Source: CAD feature listing. Evaluate the final solid. Frame: model axes, mm. Give positions to 0.01 mm unless a question says otherwise; leave off trailing zeros. Order: outer loops, then holes, each group sorted by start corner. A loop starts at its lowest first (then second) coordinate and runs counter-clockwise, first axis right, second up. Notation, with made-up numbers: (11.25, 3) - (26.25, 3) arc R13 cw to (26.25, 28) - close; hole circle Ø3 at (-7.5, 32.25). An arc over 180 degrees is marked (long way). Write each question's results on one line, items separated by ' | '. Start each with the question number.
Item 1: Mould query, pull axis X, two halves, no side actions, for faces 1 (the cylindrical face through (-2.565, 4.249, 2.465)), 2 (the flat face through (-5, 82.5, 2)), 3 (the flat face through (-9.9, 41, 2)). Classes: released by +X, released by -X, zero draft, split by the parting line, or undercut.
Item 2: Section A-A on x = -4.95. Output: boundary loops of the cut face in (y, z).
Item 3: Line query: line 1 along Y through (x, z) = (-4.95, 3.8); line 2 along Y through (x, z) = (-6.75, 3); line 3 along X through (y, z) = (4.5, 1.7). Output: solid intervals per line, ascending.
Item 4: Contact query for a flat-ended pin moving along its axis: pin 1 Ø2 at (x, y) = (-2, 39) entering from -Z. Output: stop coordinate, or through.
Item 5: Section B-B on y = 5. Output: boundary loops of the cut face in (x, z), and give its area (3 significant figures).
Item 6: Section C-C on z = 1.4. Output: boundary loops of the cut face in (x, y), and give its area (3 significant figures).
Autodesk Inventor part; units mm, degrees
ref_plane "YZ Plane" through (0, 0, 0) normal (1, 0, 0) x (0, 1, 0)
ref_plane "XZ Plane" through (0, 0, 0) normal (0, 1, 0) x (-1, 0, 0)
ref_plane "XY Plane" through (0, 0, 0) normal (0, 0, 1) x (1, 0, 0)
sketch "Sketch2" plane through (0, 0, 0) normal (0, 0, 1) x (1, 0, 0)
  line L0 (0, 0) -> (-9.9, 0)
  line L1 (-4.95, 0) -> (-4.95, 2.5)
  line L2 (-4.95, 0) -> (-2.45, 0) construction
  circle A0 centre (-4.95, 5) radius 2.5
  line L3 (-4.95, 7.5) -> (32.05, 7.5) construction
  line L4 (0, 0) -> (-9.9, 0)
  line L5 (0, 0) -> (-9.9, 0)
  line L6 (-4.95, 7.5) -> (66.05, 7.5) construction
  line L7 (-4.95, 7.5) -> (70.05, 7.5) construction
  line L8 (0, 0) -> (-9.9, 0)
  line L9 (-9.9, 0) -> (-9.9, 82.5)
  line L10 (-9.9, 82.5) -> (0, 82.5)
  line L11 (0, 82.5) -> (0, 0)
  dimension "d35" = 5
  dimension "d33" = 2.5
  dimension "d34" = 90
  dimension "d48" = 9.9
extrude "Extrusion6" add sketch "Sketch2" along normal blind 5
properties part number "Cube_Holder_SB_V1_(71mm)"
Evaluation:
1) face 1: undercut | face 2: zero draft | face 3: released by -X
2) outline: (0, 0) - (2.5, 0) - (2.5, 5) - (0, 5) - close; (7.5, 0) - (82.5, 0) - (82.5, 5) - (7.5, 5) - close
3) line 1: y = 0 to 2.5, 7.5 to 82.5 | line 2: y = 0 to 3.27, 6.73 to 82.5 | line 3: x = -9.9 to -7.4, -2.5 to 0
4) pin 1: stops at z = 0
5) outline: (-9.9, 0) - (-7.45, 0) - (-7.45, 5) - (-9.9, 5) - close; (-2.45, 0) - (0, 0) - (0, 5) - (-2.45, 5) - close | area: 24.5 mm^2
6) outline: (-9.9, 0) - (0, 0) - (0, 82.5) - (-9.9, 82.5) - close; hole circle Ø5 at (-4.95, 5) | area: 797 mm^2
